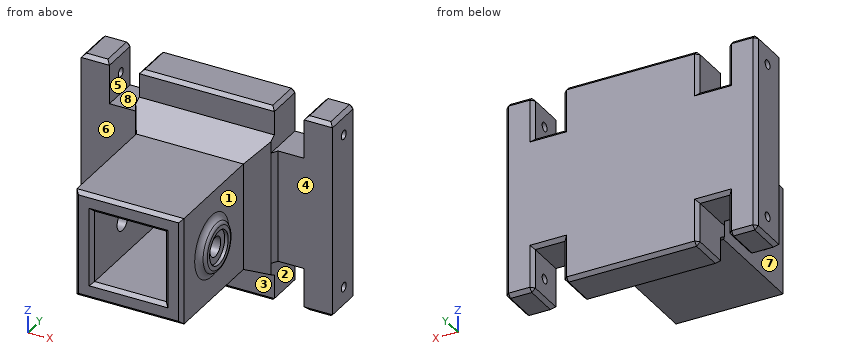
```python
from build123d import *

# Parameters (mm, degrees)
BOSS_EXTRUDE1_DEPTH = 11.5
SKETCH2_W           = 30.2
SKETCH2_H           = 30.2
SKETCH2_W_2         = 20.2
SKETCH2_H_2         = 20.2
BOSS_EXTRUDE2_DEPTH = 40
SKETCH_S_R          = 2.75
CUT_EXTRUDE1_DEPTH  = 50
BOSS_EXTRUDE3_START = 1
SKETCH_S_3_R        = 4.75
SKETCH_S_3_R_2      = 2.75
BOSS_EXTRUDE3_DEPTH = 1
BOSS_EXTRUDE4_START = 2
SKETCH_S_4_R        = 6.75
SKETCH_S_4_R_2      = 4.75
BOSS_EXTRUDE4_DEPTH = 2
FILLET1_R           = 2
FILLET2_R           = 1
CHAMFER1_START      = -15.1
CHAMFER1_DEPTH      = 30.2
CHAMFER1_START_2    = -20.1
CHAMFER1_2_DEPTH    = 40.2
CHAMFER1_START_3    = -15.8
CHAMFER1_3_DEPTH    = 31.6
CHAMFER1_START_4    = -20
CHAMFER1_4_DEPTH    = 40
SKETCH3_R           = 1.25
CUT_EXTRUDE2_DEPTH  = 10
CHAMFER2_SIZE       = 1


with BuildPart() as part:
    # Sketch1 → Boss-Extrude1 (new body)
    with BuildSketch(Plane(origin=(0, 0, 0), x_dir=(1, 0, 0), z_dir=(0, 1, 0))):
        Polygon((27.45, 15.8), (19.05, 15.8), (19.05, 27.8), (-19.05, 27.8), (-19.05, 15.8), (-27.45, 15.8), (-27.45, 27.8), (-35.45, 27.8), (-35.45, -27.8), (-27.45, -27.8), (-27.45, -15.8), (-19.05, -15.8), (-19.05, -27.8), (19.05, -27.8), (19.05, -15.8), (27.45, -15.8), (27.45, -27.8), (35.45, -27.8), (35.45, 27.8), (27.45, 27.8), align=None)
    extrude(amount=BOSS_EXTRUDE1_DEPTH)

    # Sketch2 → Boss-Extrude2 (add)
    with BuildSketch(Plane.XZ):
        Rectangle(SKETCH2_W, SKETCH2_H)
        Rectangle(SKETCH2_W_2, SKETCH2_H_2, mode=Mode.SUBTRACT)
    extrude(amount=BOSS_EXTRUDE2_DEPTH)

    # s → Cut-Extrude1 (cut)
    with BuildSketch(Plane.ZY.offset(15.1)):
        with Locations((0, -24.8)):
            Circle(SKETCH_S_R)
    extrude(amount=-CUT_EXTRUDE1_DEPTH, mode=Mode.SUBTRACT)

    # s<3> → Boss-Extrude3 (add)
    with BuildSketch(Plane.ZY.offset(15.1).offset(BOSS_EXTRUDE3_START)):
        with Locations(Location((0, -24.8, 0), (0, 0, 180))):
            Circle(SKETCH_S_3_R)
        with Locations((0, -24.8)):
            Circle(SKETCH_S_3_R_2, mode=Mode.SUBTRACT)
    boss_extrude3 = extrude(amount=-BOSS_EXTRUDE3_DEPTH)

    # s<4> → Boss-Extrude4 (add)
    with BuildSketch(Plane.ZY.offset(15.1).offset(BOSS_EXTRUDE4_START)):
        with Locations(Location((0, -24.8, 0), (0, 0, 180))):
            Circle(SKETCH_S_4_R)
        with Locations((0, -24.8)):
            Circle(SKETCH_S_4_R_2, mode=Mode.SUBTRACT)
    boss_extrude4 = extrude(amount=-BOSS_EXTRUDE4_DEPTH)

    # Mirror3: Boss-Extrude3, Boss-Extrude4 across plane
    add(boss_extrude3.mirror(Plane(origin=(0, 0, 0), x_dir=(0, 0, 1), z_dir=(1, 0, 0))))
    add(boss_extrude4.mirror(Plane(origin=(0, 0, 0), x_dir=(0, 0, 1), z_dir=(1, 0, 0))))

    # Fillet1
    fillet1_edges = [part.edges().sort_by_distance(p)[0] for p in [
        (15.1, -24.8, 6.75),
        (-15.1, -24.8, 6.75),
    ]]
    fillet(fillet1_edges, radius=FILLET1_R - 0.0001)  # a hair under: the kernel refuses the full size

    # Fillet2
    fillet2_edges = [part.edges().sort_by_distance(p)[0] for p in [
        (17.1, -24.8, 6.75),
        (-17.1, -24.8, 6.75),
    ]]
    fillet(fillet2_edges, radius=FILLET2_R)

    # Chamfer1: read off the stored shape, not the designer's step
    # Chamfer1 outline → Chamfer1 (add)
    with BuildSketch(Plane.YZ.offset(CHAMFER1_START)):
        Polygon((0, 15.8), (0, 20.1), (-8.660254038, 15.1), (0, 15.1), align=None)
        Polygon((0, -15.8), (0, -15.1), (-8.660254038, -15.1), (0, -20.1), align=None)
    extrude(amount=CHAMFER1_DEPTH)

    # Chamfer1 2 outline → Chamfer1 2 (add)
    with BuildSketch(Plane.XY.offset(CHAMFER1_START_2)):
        Polygon((19.05, -1.818653348), (19.05, 0), (15.1, 0), (15.1, -8.660254038), align=None)
        Polygon((-15.1, -8.660254038), (-15.1, 0), (-19.05, 0), (-19.05, -1.818653348), align=None)
    extrude(amount=CHAMFER1_2_DEPTH)

    # Chamfer1 3 outline → Chamfer1 3 (add)
    with BuildSketch(Plane.XY.offset(CHAMFER1_START_3)):
        Polygon((20.1, 0), (19.05, 0), (19.05, -1.818653348), align=None)
        Polygon((-19.05, -1.818653348), (-19.05, 0), (-20.1, 0), align=None)
    extrude(amount=CHAMFER1_3_DEPTH)

    # Chamfer1 4 outline → Chamfer1 4 (cut)
    with BuildSketch(Plane.YZ.offset(CHAMFER1_START_4)):
        Polygon((-8.660254038, 15.1), (0, 20.1), (-8.660254038, 20.1), align=None)
        Polygon((-8.660254038, -20.1), (0, -20.1), (-8.660254038, -15.1), align=None)
    extrude(amount=CHAMFER1_4_DEPTH, mode=Mode.SUBTRACT)

    # Sketch3 → Cut-Extrude2 (cut)
    with BuildSketch(Plane(origin=(35.45, 0, 0), x_dir=(0, 0, -1), z_dir=(1, 0, 0))):
        with Locations((-21.8, 5.75)):
            Circle(SKETCH3_R)
        with Locations((21.8, 5.75)):
            Circle(SKETCH3_R)
    cut_extrude2 = extrude(amount=-CUT_EXTRUDE2_DEPTH, mode=Mode.SUBTRACT)

    # Mirror4: Cut-Extrude2 across plane
    add(cut_extrude2.mirror(Plane(origin=(0, 0, 0), x_dir=(0, 0, 1), z_dir=(1, 0, 0))), mode=Mode.SUBTRACT)

    # Chamfer2
    chamfer2_edges = [part.edges().sort_by_distance(p)[0] for p in [
        (31.45, 11.5, -27.8),
        (27.45, 11.5, -21.8),
        (0, 0, 27.8),
        (23.25, 11.5, -15.8),
        (-31.45, 0, 27.8),
        (-31.45, 0, -27.8),
        (19.05, 11.5, -21.8),
        (0, 0, -27.8),
        (31.45, 0, -27.8),
        (31.45, 0, 27.8),
        (0, 11.5, -27.8),
        (-19.05, 11.5, -21.8),
        (27.45, 5.75, 27.8),
        (19.05, 5.75, 27.8),
        (-19.05, 5.75, 27.8),
        (-27.45, 5.75, 27.8),
        (-35.45, 5.75, 27.8),
        (-35.45, 5.75, -27.8),
        (-27.45, 5.75, -27.8),
        (-23.25, 11.5, -15.8),
        (-19.05, 5.75, -27.8),
        (19.05, 5.75, -27.8),
        (27.45, 5.75, -27.8),
        (35.45, 5.75, -27.8),
        (35.45, 5.75, 27.8),
        (-27.45, 11.5, -21.8),
        (-31.45, 11.5, -27.8),
        (-35.45, 11.5, 0),
        (31.45, 11.5, 27.8),
        (-31.45, 11.5, 27.8),
        (-27.45, 11.5, 21.8),
        (-23.25, 11.5, 15.8),
        (-19.05, 11.5, 21.8),
        (15.1, -40, 0),
        (0, -40, 15.1),
        (-15.1, -40, 0),
        (0, -40, -15.1),
        (0, 11.5, 27.8),
        (10.1, -40, 0),
        (0, -40, 10.1),
        (-10.1, -40, 0),
        (0, -40, -10.1),
        (19.05, 11.5, 21.8),
        (23.25, 11.5, 15.8),
        (27.45, 11.5, 21.8),
        (35.45, 11.5, 0),
    ]]
    chamfer(chamfer2_edges, length=CHAMFER2_SIZE)


solid = part.part
```
For this review, take the finished solid that the model builds, in its own axes (mm). Face numbers are marked on the shaded views. A direction names the side the tool comes from. Give positions to 0.01 mm unless a question says otherwise; leave off trailing zeros. Write each loop counter-clockwise with the first axis right and the second up, starting at its lowest first coordinate (ties: lowest second). Pieces come first, ordered by that corner, then holes.
Item 1: The part is to be moulded in two halves that separate along X. For the marked faces 6, 7 and 8, say which applies: +X half, -X half, draft (parallel to the pull), parting line (faces both ways), or undercut.
Item 2: Take a section at A-A (z = -21.8). Give the boundary of the cut face in (x, y).
Item 3: Take a section at B-B (y = -15). Give the boundary of the cut face in (x, z).
Item 4: Take a section at C-C (x = -7.5). Give the boundary of the cut face in (y, z), and give its area (3 significant figures).
Item 5: Machinability: for the marked faces 1, 2, 3, 4 and 5, which of the approach directions +Z, -Z, +X, -X, +Y, -Y give a long, thin tool a straight path to every point of the face, cutting with its end or side? Answer none if there is none.
Item 6: Wall thickness on probe 1 along X at (y, z) = (9.5, -17.5); probe 2 along Z at (x, y) = (-32.5, 5.75); probe 3 along X at (y, z) = (-12.5, -3): over which ranges is each line inside the solid? List them lowest first.
Item 7: Insertion check: P1, Ø16, axis at x = 5, y = -11, coming from the -Z side; P2, Ø1, axis at x = -16, z = 2, coming from the -Y side; P3, Ø12.5, axis at x = -26.5, z = -5.5, coming from the -Y side; P4, Ø3, axis at y = -25.5, z = 0.5, coming from the +X side. Each pin has a flat end and moves straight along its axis. Give the tip position at first contact, or say it passes through.
Item 8: Take a section at D-D (x = -30.5). Give the boundary of the cut face in (y, z).
Established:
1. face 6: draft
1. face 7: -X half
1. face 8: undercut
2. outline: (-35.45, 0) - (-27.45, 0) - (-27.45, 4.5) - (-35.45, 4.5) - close; (-35.45, 7) - (-27.45, 7) - (-27.45, 10.5) - (-28.45, 11.5) - (-34.45, 11.5) - (-35.45, 10.5) - close; (-19.05, 0) - (19.05, 0) - (19.05, 10.5) - (18.05, 11.5) - (-18.05, 11.5) - (-19.05, 10.5) - close; (27.45, 0) - (35.45, 0) - (35.45, 4.5) - (27.45, 4.5) - close; (27.45, 7) - (35.45, 7) - (35.45, 10.5) - (34.45, 11.5) - (28.45, 11.5) - (27.45, 10.5) - close
3. outline: (-15.1, -15.1) - (15.1, -15.1) - (15.1, 15.1) - (-15.1, 15.1) - close; hole (-10.1, -10.1) - (10.1, -10.1) - (10.1, 10.1) - (-10.1, 10.1) - close
4. outline: (-40, -14.1) - (-39, -15.1) - (-8.66, -15.1) - (0, -20.1) - (0, -26.8) - (1, -27.8) - (10.5, -27.8) - (11.5, -26.8) - (11.5, 26.8) - (10.5, 27.8) - (1, 27.8) - (0, 26.8) - (0, 20.1) - (-8.66, 15.1) - (-39, 15.1) - (-40, 14.1) - (-40, 11.1) - (-39, 10.1) - (0, 10.1) - (0, -10.1) - (-39, -10.1) - (-40, -11.1) - close
4. area: 1,080 mm2
5. face 1: +X
5. face 2: -Z, +Y, -Y
5. face 3: -Z, +X, -X, -Y
5. face 4: +Z, -Z, +X, -Y
5. face 5: +Z, +Y, -Y
6. probe 1: x = -35.45 to -27.45, -19.05 to 19.05, 27.45 to 35.45
6. probe 2: z = -27.8 to -23.05, -20.55 to 20.55, 23.05 to 27.8
6. probe 3: x = -15.1 to -10.1, 10.1 to 15.1
7. P1: stops at z = -18.37
7. P2: stops at y = -32.09
7. P3: stops at y = 0
7. P4: passes through
8. outline: (0, -26.8) - (1, -27.8) - (10.5, -27.8) - (11.5, -26.8) - (11.5, 26.8) - (10.5, 27.8) - (1, 27.8) - (0, 26.8) - close; hole circle Ø2.5 at (5.75, -21.8); hole circle Ø2.5 at (5.75, 21.8)
